Could you check a few things on this model? Use its own coordinates, in mm. A direction names the side the tool comes from. Coordinates: 2 decimals unless noted, no trailing zeros. Loops run counter-clockwise (first coordinate to the right, second up) from the corner with the lowest first, then second, coordinate; pieces in that order, holes last. Notation, with made-up numbers: (5.5, 26) - (14.5, 26) arc R23 cw to (14.5, 36) - close; hole circle Ø5 at (84.5, 30.25). An arc over 180 degrees is marked (long way). Use CSV: the item, a comma, the result in double quotes.
from build123d import *

# Parameters (mm, degrees)
SKETCH_1_W                     = 52
SKETCH_1_H                     = 44
EXTRUDE_1_DEPTH                = 16.5
SHELL_1_T                      = -1.8
CUT_EXTRUDE_1_DEPTH            = 68.500296296
CUT_EXTRUDE_1_DEPTH_BACK       = 68.500296296
SKETCH_3_W                     = 40.4
SKETCH_3_H                     = 14.7
SKETCH_4_W                     = 12.5
SKETCH_4_H                     = 40.4
EXTRUDE_2_DEPTH                = 1.5
CUT_EXTRUDE_2_DEPTH            = 1
EXTRUDE_3_REACH                = 66.438
SKETCH_6_R                     = 1.75
HOLE_WIZARD_M1_6_1_D           = 1.25
HOLE_WIZARD_M1_6_1_DEPTH       = 12
HOLE_WIZARD_M1_6_1_CSINK_D     = 1.65
HOLE_WIZARD_M1_6_1_CSINK_ANGLE = 90
HOLE_WIZARD_M1_6_1_TIP         = 0.375537887
SKETCH_11_W                    = 22
SKETCH_11_H                    = 22
CUT_EXTRUDE_3_DEPTH            = 1.3
CHAMFER_2_SIZE                 = 0.6
FILLET_1_R                     = 1
SKETCH_13_W                    = 9.6
SKETCH_13_H                    = 1.8
EXTRUDE_4_DEPTH                = 1.2
CHAMFER_3_SIZE                 = 2.3
SKETCH_14_R                    = 3
CUT_EXTRUDE_5_DEPTH            = 16


with BuildPart() as part:
    # 스케치1 → 보스-돌출1 (new body)
    with BuildSketch(Plane(origin=(0, 0, 0), x_dir=(1, 0, 0), z_dir=(0, 1, 0))):
        with Locations((20, 20)):
            Rectangle(SKETCH_1_W, SKETCH_1_H)
    extrude(amount=-EXTRUDE_1_DEPTH)

    # 쉘1
    shell_1_openings = [part.faces().sort_by_distance(p)[0] for p in [
        (20, 0, -20),
    ]]
    offset(amount=SHELL_1_T, openings=shell_1_openings, kind=Kind.INTERSECTION)

    # 스케치3 → 컷-돌출1 (cut, two sides: drawn at the far end of the back side and taken through both)
    with BuildSketch(Plane(origin=(-4.2, 0, 0), x_dir=(0, 0, -1), z_dir=(1, 0, 0)).offset(-CUT_EXTRUDE_1_DEPTH_BACK)):
        with Locations((20, -7.35)):
            Rectangle(SKETCH_3_W, SKETCH_3_H)
    extrude(amount=CUT_EXTRUDE_1_DEPTH + CUT_EXTRUDE_1_DEPTH_BACK, mode=Mode.SUBTRACT)

    # 스케치4 → 보스-돌출2 (add)
    with BuildSketch(Plane(origin=(0, -14.7, 0), x_dir=(1, 0, 0), z_dir=(0, 1, 0))):
        with Locations((39.75, 20)):
            Rectangle(SKETCH_4_W, SKETCH_4_H)
        with Locations((0.25, 20)):
            Rectangle(SKETCH_4_W, SKETCH_4_H)
    extrude(amount=EXTRUDE_2_DEPTH)

    # 스케치5 → 컷-돌출2 (cut)
    with BuildSketch(Plane(origin=(0, -13.2, 0), x_dir=(1, 0, 0), z_dir=(0, 1, 0))):
        Polygon((2.34, -0.2), (1.34, -0.2), (1.34, 40.2), (2.34, 40.2), (4.34, 40.2), (9.34, 40.2), (9.34, -0.2), (4.34, -0.2), align=None)
        Polygon((35.66, 40.2), (37.66, 40.2), (38.66, 40.2), (38.66, -0.2), (37.66, -0.2), (35.66, -0.2), (30.66, -0.2), (30.66, 40.2), align=None)
    extrude(amount=-CUT_EXTRUDE_2_DEPTH, mode=Mode.SUBTRACT)

    # 스케치6 → 보스-돌출3 (add, up to next)
    with BuildSketch(Plane(origin=(0, 0, 0), x_dir=(1, 0, 0), z_dir=(0, 1, 0)), mode=Mode.PRIVATE) as extrude_3_sk1:
        with Locations((7.5, 0)):
            Circle(SKETCH_6_R)
    extrude_3_tool1 = extrude(extrude_3_sk1.sketch, amount=-EXTRUDE_3_REACH, mode=Mode.PRIVATE) - part.part
    # 스케치6 → 보스-돌출3 (add, up to next)
    with BuildSketch(Plane(origin=(0, 0, 0), x_dir=(1, 0, 0), z_dir=(0, 1, 0)), mode=Mode.PRIVATE) as extrude_3_sk2:
        with Locations((7.5, 40)):
            Circle(SKETCH_6_R)
    extrude_3_tool2 = extrude(extrude_3_sk2.sketch, amount=-EXTRUDE_3_REACH, mode=Mode.PRIVATE) - part.part
    # 스케치6 → 보스-돌출3 (add, up to next)
    with BuildSketch(Plane(origin=(0, 0, 0), x_dir=(1, 0, 0), z_dir=(0, 1, 0)), mode=Mode.PRIVATE) as extrude_3_sk3:
        with Locations((32.5, 40)):
            Circle(SKETCH_6_R)
    extrude_3_tool3 = extrude(extrude_3_sk3.sketch, amount=-EXTRUDE_3_REACH, mode=Mode.PRIVATE) - part.part
    # 스케치6 → 보스-돌출3 (add, up to next)
    with BuildSketch(Plane(origin=(0, 0, 0), x_dir=(1, 0, 0), z_dir=(0, 1, 0)), mode=Mode.PRIVATE) as extrude_3_sk4:
        with Locations((32.5, 0)):
            Circle(SKETCH_6_R)
    extrude_3_tool4 = extrude(extrude_3_sk4.sketch, amount=-EXTRUDE_3_REACH, mode=Mode.PRIVATE) - part.part
    add(extrude_3_tool1.solids().sort_by_distance((7.5, 0, 0))[0])
    add(extrude_3_tool2.solids().sort_by_distance((7.5, 0, -40))[0])
    add(extrude_3_tool3.solids().sort_by_distance((32.5, 0, -40))[0])
    add(extrude_3_tool4.solids().sort_by_distance((32.5, 0, 0))[0])

    # M1.6 나사 구멍1
    with Locations(Plane(origin=(0, 0, 0), x_dir=(1, 0, 0), z_dir=(0, 1, 0))):
        with Locations((7.5, 0), (32.5, 0), (7.5, 40), (32.5, 40)):
            CounterSinkHole(HOLE_WIZARD_M1_6_1_D / 2, HOLE_WIZARD_M1_6_1_CSINK_D / 2, depth=HOLE_WIZARD_M1_6_1_DEPTH, counter_sink_angle=HOLE_WIZARD_M1_6_1_CSINK_ANGLE)
            with Locations((0, 0, -(HOLE_WIZARD_M1_6_1_DEPTH + HOLE_WIZARD_M1_6_1_TIP / 2))):  # 118° drill point
                Cone(0, HOLE_WIZARD_M1_6_1_D / 2, HOLE_WIZARD_M1_6_1_TIP, mode=Mode.SUBTRACT)

    # 스케치11 → 컷-돌출3 (cut)
    with BuildSketch(Plane(origin=(0, -14.7, 0), x_dir=(1, 0, 0), z_dir=(0, 1, 0))):
        with Locations((20, 20)):
            Rectangle(SKETCH_11_W, SKETCH_11_H)
    extrude(amount=-CUT_EXTRUDE_3_DEPTH, mode=Mode.SUBTRACT)

    # 모따기2
    chamfer_2_edges = [part.edges().sort_by_distance(p)[0] for p in [
        (20, -16.5, -42),
        (20, -16.5, 2),
        (-6, -8.25, -42),
        (46, -8.25, -42),
        (46, -8.25, 2),
        (-6, -8.25, 2),
    ]]
    chamfer(chamfer_2_edges, length=CHAMFER_2_SIZE)

    # 필렛1
    fillet_1_edges = [part.edges().sort_by_distance(p)[0] for p in [
        (38.66, -13.7, 0.2),
        (38.66, -13.7, -40.2),
        (9.238533865, -7.35, 0.2),
        (6.5, -14.45, -1.436140662),
        (5.761466135, -7.1, 0.2),
        (5.761466135, -7.1, -40.2),
        (6.5, -14.45, -38.563859338),
        (9.238533865, -7.35, -40.2),
        (30.761466135, -7.35, -40.2),
        (33.5, -14.45, -38.563859338),
        (34.238533865, -7.1, -40.2),
        (34.238533865, -7.1, 0.2),
        (33.5, -14.45, -1.436140662),
        (30.761466135, -7.35, 0.2),
        (9, -15.35, -9),
        (9, -15.35, -31),
        (31, -15.35, -31),
        (31, -15.35, -9),
        (1.34, -13.7, -40.2),
        (1.34, -13.7, 0.2),
    ]]
    fillet(fillet_1_edges, radius=FILLET_1_R)

    # 스케치13 → 보스-돌출4 (add)
    with BuildSketch(Plane(origin=(0, 0, 0), x_dir=(1, 0, 0), z_dir=(0, 1, 0))):
        with Locations((20, 41.1)):
            Rectangle(SKETCH_13_W, SKETCH_13_H)
    extrude(amount=EXTRUDE_4_DEPTH)

    # 모따기3
    # the kernel refuses this chamfer: 2.3 mm, written as the material it takes off along each edge
    with BuildSketch(Plane(origin=(46, -16.5, 7.314870872), x_dir=(0.027495876610586976, 0.9996219169112968, 0), z_dir=(0, 0, -1))) as chamfer_3_piece_1:
        Polygon((CHAMFER_3_SIZE * 0.999621916911, -CHAMFER_3_SIZE * 0.0274958766106), (-CHAMFER_3_SIZE * 0.0274958766106, -CHAMFER_3_SIZE * 0.999621916911), (0, 0), align=None)
    extrude(amount=54.629741745, mode=Mode.SUBTRACT)
    with BuildSketch(Plane(origin=(-6, -16.5, -47.314870872), x_dir=(0.9996219169112966, -0.027495876610586965, 0), z_dir=(0, 0, 1))) as chamfer_3_piece_2:
        Polygon((CHAMFER_3_SIZE * 0.999621916911, CHAMFER_3_SIZE * 0.0274958766106), (-CHAMFER_3_SIZE * 0.0274958766106, CHAMFER_3_SIZE * 0.999621916911), (0, 0), align=None)
    extrude(amount=54.629741745, mode=Mode.SUBTRACT)

    # 스케치14 → 컷-돌출5 (cut)
    with BuildSketch(Plane(origin=(0, 0, 0), x_dir=(1, 0, 0), z_dir=(0, 1, 0))):
        with Locations(Location((2.34, 20, 0), (0, 0, 270))):
            Circle(SKETCH_14_R)
        with Locations(Location((37.66, 20, 0), (0, 0, 270))):
            Circle(SKETCH_14_R)
    extrude(amount=-CUT_EXTRUDE_5_DEPTH, mode=Mode.SUBTRACT)


solid = part.part
(1) Which directions (+Z, -Z, +X, -X, +Y, -Y) give clear straight access to the entire face, cutting with the end or side of a thin tool? Please do faces 1 (the face through (35, 0, -41)), 2 (the face through (32.164, -6.183, -40.527)), 3 (the face through (20, -16.5, -20)).
Computed:
face 1,"+Z, -Z, +X, +Y"
face 2,"+Y"
face 3,"+Z, -Z, +X, -X, -Y"
(2) Suppose I cut it at B-B (x = 28). Write out the boundary of the cut face in (y, z).
Computed:
outline,"(-16.5, -41.4) - (-15.9, -42) - (0, -42) - (0, -40.2) - (-14.7, -40.2) - (-14.7, -31) - (-16, -31) - (-16, -9) - (-14.7, -9) - (-14.7, 0.2) - (0, 0.2) - (0, 2) - (-15.9, 2) - (-16.5, 1.4) - close"
(3) Suppose I cut it at D-D (z = -34). Write out the boundary of the cut face in (x, y).
Computed:
outline,"(-6, -14.2) - (-3.7, -16.5) - (43.7, -16.5) - (46, -14.2) - (46, -13.2) - (38.66, -13.2) - (38.66, -14.2) - (33.5, -14.2) - (33.5, -14.7) - (6.5, -14.7) - (6.5, -14.2) - (1.34, -14.2) - (1.34, -13.2) - (-6, -13.2) - close"
(4) Suppose I cut it at C-C (z = -16). Write out the boundary of the cut face in (x, y), plus the area to 3 significant figures.
Computed:
outline,"(-6, -14.2) - (-3.7, -16.5) - (43.7, -16.5) - (46, -14.2) - (46, -13.2) - (38.66, -13.2) - (38.66, -14.2) - (33.5, -14.2) - (33.5, -14.7) - (31, -14.7) - (31, -16) - (9, -16) - (9, -14.7) - (6.5, -14.7) - (6.5, -14.2) - (1.34, -14.2) - (1.34, -13.2) - (-6, -13.2) - close"
area,"86.9 mm²"
(5) Thinking about a two-plate mould opening in X: for faces 4 (the face through (32.53, -7.25, -1.75)), 5 (the face through (20, 1.2, -41)), which applies, +X half, -X half, draft (parallel to the pull), parting line (faces both ways), or undercut?
Computed:
face 4,"undercut"
face 5,"draft"
(6) Suppose I cut it at A-A (y = -4.75). State how many separate pieces and enclosed holes the cut face has, plus the area to 3 significant figures.
Computed:
separate pieces,"2"
enclosed holes,"4"
area,"205 mm²"
(7) Will these pins go through, and if not, where does the flat tip stop? pin 1 (1 mm diameter, centred on x = 32.5, z = 0, fed in from +Y); pin 2 (4 mm diameter, centred on x = 2.5, z = -40.5, fed in from +Y); pin 3 (1.3 mm diameter, centred on y = 0.5, z = -41.5, fed in from +X); pin 4 (1.4 mm diameter, centred on y = -15.5, z = -21, fed in from -X).
Computed:
pin 1,"stops at y = -12.08"
pin 2,"stops at y = 0"
pin 3,"stops at x = 46"
pin 4,"stops at x = -5.4"
(8) Please list where these lines run through material, in increasing order: line 1 (Z direction, x = 7.5, y = -7.5) (3 decimals); line 2 (Z direction, x = 19, y = -8.25); line 3 (X direction, y = -3, z = -40) (3 decimals).
Computed:
line 1,"z = -42 to -40.625, -39.375 to -38.25, -1.75 to -0.625, 0.625 to 2"
line 2,"z = -42 to -40.2, 0.2 to 2"
line 3,"x = 5.469 to 6.875, 8.125 to 9.531, 30.469 to 31.875, 33.125 to 34.531"
